```python
from build123d import *

# Parameters (mm, degrees)
SKETCH1_R           = 6
BOSS_EXTRUDE1_DEPTH = 30
SKETCH1_3_R         = 6
BOSS_EXTRUDE2_DEPTH = 15
BOSS_EXTRUDE3_DEPTH = 6
SKETCH2_3_R         = 23
SKETCH2_3_R_2       = 14
BOSS_EXTRUDE4_DEPTH = 16
FILLET1_R           = 6


with BuildPart() as part:
    # Sketch1 → Boss-Extrude1 (new body)
    with BuildSketch(Plane(origin=(0, 0, 0), x_dir=(1, 0, 0), z_dir=(0, 1, 0))):
        with BuildLine():
            ThreePointArc((79.052558883, -11), (82, 0), (79.052558883, 11))
            Line((79.052558883, 11), (60, 11))
            ThreePointArc((60, 11), (49, 0), (60, -11))
            Line((60, -11), (79.052558883, -11))
        make_face()
        with Locations((60, 0)):
            Circle(SKETCH1_R, mode=Mode.SUBTRACT)
    extrude(amount=BOSS_EXTRUDE1_DEPTH)

    # Sketch1_3 → Boss-Extrude2 (add)
    with BuildSketch(Plane(origin=(0, 0, 0), x_dir=(1, 0, 0), z_dir=(0, 1, 0))):
        with BuildLine():
            Line((0, 62), (0, -62))
            ThreePointArc((0, -62), (3.352861242, -61.522079738), (6.438655763, -60.126386916))
            Line((6.438655763, -60.126386916), (71.804202232, -18.565042679))
            ThreePointArc((71.804202232, -18.565042679), (82, 0), (71.804202232, 18.565042679))
            Line((71.804202232, 18.565042679), (6.438655763, 60.126386916))
            ThreePointArc((6.438655763, 60.126386916), (3.352861242, 61.522079738), (0, 62))
        make_face()
        with Locations((60, 0)):
            Circle(SKETCH1_3_R, mode=Mode.SUBTRACT)
    extrude(amount=BOSS_EXTRUDE2_DEPTH)

    # Sketch2 → Boss-Extrude3 (add)
    with BuildSketch(Plane.ZY):
        with BuildLine():
            Line((44, 15), (21.543109519, 75.055708054))
            ThreePointArc((21.543109519, 75.055708054), (22.632846915, 71.093194417), (23, 67))
            ThreePointArc((23, 67), (-4.093194417, 44.367153085), (-21.543109519, 75.055708054))
            Line((-21.543109519, 75.055708054), (-44, 15))
            Line((-44, 15), (44, 15))
        make_face()
    extrude(amount=-BOSS_EXTRUDE3_DEPTH)

    # Sketch2_3 → Boss-Extrude4 (add)
    with BuildSketch(Plane.ZY):
        with Locations((0, 67)):
            Circle(SKETCH2_3_R)
        with Locations((0, 67)):
            Circle(SKETCH2_3_R_2, mode=Mode.SUBTRACT)
    extrude(amount=-BOSS_EXTRUDE4_DEPTH)

    # Fillet1
    fillet1_edges = [part.edges().sort_by_distance(p)[0] for p in [
        (3, 15, 44),
        (3, 15, -44),
    ]]
    fillet(fillet1_edges, radius=FILLET1_R)

    # Mirror1: part across plane


with BuildPart() as part_1:
    add(part.part)
    add(part.part.mirror(Plane(origin=(0, 15, 0), x_dir=(0, 0, 1), z_dir=(1, 0, 0))))


solid = part_1.part
```
Input: part model. Units: mm. Frame: model coordinates. A direction names the side the tool comes from. Give positions to 0.01 mm unless a question says otherwise; leave off trailing zeros. Order: outer loops, then holes, each group sorted by start corner. A loop starts at its lowest first (then second) coordinate and runs counter-clockwise, first axis right, second up. Notation, with made-up numbers: M 82.5,-17 L 88.5,-17 A17 ccw 88.5,0 Z; hole C -7.5,-26 d11. An arc over 180 degrees is marked long. One line per question, with ' | ' between items. Start each with the question number.
1. Pull-direction query (Z, two-part tool) for faces 6 (the face through (-54, 15, 0)), 7 (the face through (-0.1, 16.1, -44.7)), 8 (the face through (69, 22, 11)), 9 (the face through (-6, 32, -1)); classes: released by +Z, released by -Z, zero draft, split by the parting line, or undercut.
2. Access query for faces 1 (the face through (16, 52, 0)), 2 (the face through (-16, 52, 0)), 3 (the face through (0.224, 89.804, -2.994)), 4 (the face through (70, 22, -11)), 5 (the face through (-69, 22, 11)). Directions: +Z, -Z, +X, -X, +Y, -Y. A direction counts if a zero-diameter tool reaches every point of the face in a straight line with its end or side. Return the directions, or none.
3. First-contact query: pin 1 Ø4.5 at (x, y) = (-66.5, 24.5) entering from +Z; pin 2 Ø1 at (y, z) = (27, 33.5) entering from +X; pin 3 Ø1.5 at (x, y) = (11, 14) entering from -Z. Flat tips, straight axial feed; report the tip coordinate or a pass-through.
4. Section query A-A (z = 0). Return the cut outline in (x, y).
5. Section query D-D (x = 51.5). Return the cut outline in (y, z), and give its area (3 significant figures).
6. Material intervals for probe 1 along X at (y, z) = (9.25, 0); probe 2 along X at (y, z) = (19, 0); probe 3 along Z at (x, y) = (60, 24), sorted ascending. Write a range as [from, to].
7. Section query B-B (y = 6.5). Return the cut outline in (x, z), and give its area (3 significant figures).
8. Section query C-C (y = 78). Return the cut outline in (x, z), and give its area (3 significant figures).
Here are the results:
1) face 6: undercut | face 7: released by -Z | face 8: released by +Z | face 9: zero draft
2) face 1: +Z, -Z, +X, +Y | face 2: +Z, -Z, -X, +Y | face 3: none | face 4: -Z, +X, +Y | face 5: +Z, -X, +Y
3) pin 1: z = 11 | pin 2: x = 6 | pin 3: z = -57.7
4) outline: M -82,0 L -66,0 L -66,30 L -82,30 Z; M -54,0 L 54,0 L 54,30 L 49,30 L 49,15 L 6,15 L 6,44 L 16,44 L 16,53 L -16,53 L -16,44 L -6,44 L -6,15 L -49,15 L -49,30 L -54,30 Z; M -16,81 L 16,81 L 16,90 L -16,90 Z; M 66,0 L 82,0 L 82,30 L 66,30 Z
5) outline: M 0,-31.48 L 15,-31.48 L 15,-6.98 L 30,-6.98 L 30,6.98 L 15,6.98 L 15,31.48 L 0,31.48 Z | area: 1,150 mm²
6) probe 1: [-82, -66], [-54, 54], [66, 82] | probe 2: [-82, -66], [-54, -49], [-6, 6], [49, 54], [66, 82] | probe 3: [-11, -6], [6, 11]
7) outline: M -71.8,-18.57 L -6.44,-60.13 A12 ccw 6.44,-60.13 L 71.8,-18.57 A22 ccw 71.8,18.57 L 6.44,60.13 A12 ccw -6.44,60.13 L -71.8,18.57 A22 ccw Z; hole C -60,0 d12; hole C 60,0 d12 | area: 12,200 mm²
8) outline: M -16,-20.2 L 16,-20.2 L 16,-8.66 L -16,-8.66 Z; M -16,8.66 L 16,8.66 L 16,20.2 L -16,20.2 Z | area: 738 mm²
